Check sheet for the modelled part. Datum: model origin and axes. Units: mm. Face numbers are marked on the shaded views. A direction names the side the tool comes from. Round coordinates to 2 decimals unless told otherwise and drop trailing zeros. Write each loop counter-clockwise with the first axis right and the second up, starting at its lowest first coordinate (ties: lowest second). Pieces come first, ordered by that corner, then holes. Notation, with made-up numbers: (-10.5, 18) -> (8.5, 18) arc R37 cw to (8.5, 54) -> close; hole circle Ø6 at (48.5, 51). An arc over 180 degrees is marked (long way). Write item = value, one per line.
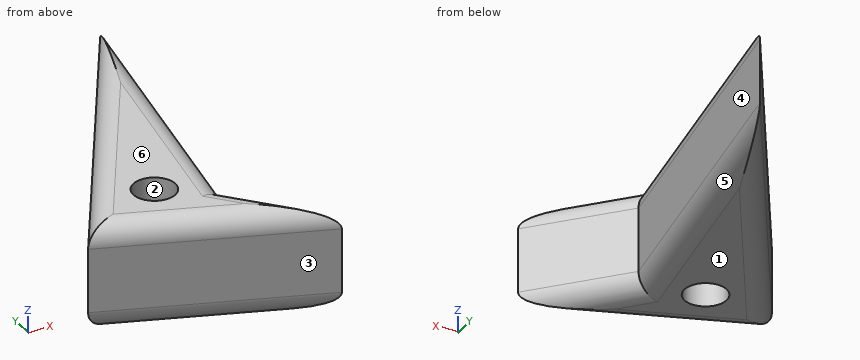
from build123d import *

# Parameters (mm, degrees)
F1_DEPTH = 12.7
F2_R     = 2.54
F3_R     = 2.54
F4_R     = 2.5016114836
F5_DEPTH = 12.954


with BuildPart() as f1:
    # F0 (on Top) → F1 (new body)
    with BuildSketch(Plane.XY):
        Polygon((-2.0137657411, 54.22963202), (-25.2730008215, 15.8750005066), (-8.7629994377, 16.6370011866), align=None)
        Polygon((-8.7629994377, 16.6370011866), (-25.2730008215, 15.8750005066), (0, 6.5225157887), align=None)
    extrude(amount=F1_DEPTH)

    # F2
    f2_edges = [f1.edges().sort_by_distance(p)[0] for p in [
        (-13.643383, 35.052316, 12.7),
        (-12.6365, 11.198758, 12.7),
        (-4.3815, 11.579758, 12.7),
        (-5.388383, 35.433317, 12.7),
    ]]
    fillet(f2_edges, radius=F2_R)

    # F3
    f3_edges = [f1.edges().sort_by_distance(p)[0] for p in [
        (-13.643383, 35.052316, 0),
        (-12.6365, 11.198758, 0),
        (-4.3815, 11.579758, 0),
        (-5.388383, 35.433317, 0),
    ]]
    fillet(f3_edges, radius=F3_R)

    # F4 (on face) → F5 (cut)
    with BuildSketch(Plane.XY.offset(12.7)):
        with Locations((-15.1129998267, 19.6850001812)):
            Circle(F4_R)
    extrude(amount=-F5_DEPTH, mode=Mode.SUBTRACT)


solid = f1.part
(1) Release check for a two-part mould opening along Y. For the marked faces 1, 2 and 3 record: pulls with the +Y half, pulls with the -Y half, needs draft (parallel to the pull), parting line crosses it, or undercut.
Worked answers:
face_1 = needs draft
face_2 = undercut
face_3 = pulls with the -Y half
(2) Sectioned sample at B-B on z = 1.25. Enter the section's corners in (x, y) (3 decimals), then the cut area to 3 significant figures.
Worked answers:
outline = (-24.751, 16.057) -> (-1.164, 7.329) -> (-9.139, 16.534) -> (-2.695, 52.428) -> close; hole circle Ø5.003 at (-15.113, 19.685)
area = 333 mm²
(3) Access from +Z, -Z, +X, -X, +Y, -Y to the whole of each face (thin tool, end or side, straight path). Record for the marked faces 4, 5 and 6.
Worked answers:
face_4 = +Z, -Z, +X
face_5 = -Z, +X
face_6 = +Z, +X, -X, +Y, -Y
(4) Go/stop test with flat-tipped pins: P1, Ø2, axis at x = -15, y = 33, coming from the -Z side; P2, Ø6, axis at x = -22.5, z = 10.5, coming from the +Y side; P3, Ø1.5, axis at x = -3.5, z = 9.5, coming from the +Y side; P4, Ø4.5, axis at x = -15.113, y = 19.685, coming from the +Z side. Record where each tip stops, or that it passes through.
Worked answers:
P1 = 0.6
P2 = 25.38
P3 = 53.02
P4 = through
(5) Material ranges on L1, parallel to Y at x = -17, z = 11.75; L2, parallel to Y at x = -21.5, z = 3.5; L3, parallel to X at y = 19, z = 11.75, recorded low to high. Write a range as [from, to].
Worked answers:
L1 = [13.41, 18.04], [21.33, 28.44]
L2 = [14.48, 22.1]
L3 = [-22.72, -17.52], [-12.71, -8.91]
(6) Sectioned sample at A-A on z = 6. Enter the section's corners in (x, y) (3 decimals).
Worked answers:
outline = (-25.273, 15.875) -> (0, 6.523) -> (-8.763, 16.637) -> (-2.014, 54.23) -> close; hole circle Ø5.003 at (-15.113, 19.685)
